Autodesk Inventor part; units mm, degrees
ref_plane "YZ Plane" through (0, 0, 0) normal (1, 0, 0) x (0, 1, 0)
ref_plane "XZ Plane" through (0, 0, 0) normal (0, 1, 0) x (-1, 0, 0)
ref_plane "XY Plane" through (0, 0, 0) normal (0, 0, 1) x (1, 0, 0)
sketch "Sketch1" plane through (0, 0, 0) normal (0, 0, 1) x (1, 0, 0)
  line L0 (-129.1, 49.6) -> (111.9, 49.6)
  line L1 (111.9, 49.6) -> (111.9, -75.4)
  line L2 (111.9, -75.4) -> (-129.1, -75.4)
  line L3 (-129.1, -75.4) -> (-129.1, 49.6)
  line L4 (-116.8, -67) -> (-68.1, -67)
  line L5 (-45.7, -67) -> (3, -67)
  line L6 (3, 18.4) -> (-45.7, 18.4)
  line L7 (-116.8, 18.5) -> (-68.1, 18.5)
  line L8 (-120.7, 14.5) -> (-120.7, -63.1)
  line L9 (-120.7, -67) -> (7.3759, -67) construction
  line L10 (7.3759, -67) -> (7.3759, 18.4) construction
  line L11 (7.3759, 18.4) -> (-120.7, 18.4) construction
  line L12 (-120.7, 18.4) -> (-120.7, -67) construction
  line L13 (4.7803, -64.4044) -> (-118.1044, -64.4044)
  line L14 (-118.1044, -64.4044) -> (-118.1044, 15.8044)
  line L15 (-118.1044, 15.8044) -> (4.7803, 15.8044)
  line L16 (4.7803, 15.8044) -> (4.7803, -64.4044)
  line L17 (-129.1, -55.4) -> (-129.1, -65.4)
  line L18 (-129.1, -75.4) -> (-119.1, -75.4) construction
  line L19 (111.9, -72.4764) -> (111.9, -32.5764) construction
  dimension "d78" = 0
extrude "Extrusion1" add sketch "Sketch1" along normal blind 2
sketch "Sketch10" plane through (0, 0, 0) normal (0, 0, -1) x (-1, 0, 0)
  line L0 (129.1, 49.6) -> (-111.9, 49.6)
  line L1 (-111.9, 49.6) -> (-111.9, -75.4)
  line L2 (-111.9, -75.4) -> (129.1, -75.4)
  line L3 (129.1, -75.4) -> (129.1, 49.6)
  line L4 (-104.9, -68.4) -> (-104.9, 42.6)
  line L5 (-104.9, 42.6) -> (122.1, 42.6)
  line L6 (122.1, 42.6) -> (122.1, -68.4)
  line L7 (122.1, -68.4) -> (-104.9, -68.4)
  line L8 (-3, 18.4) -> (45.7, 18.4)
  line L9 (-6.9, -63.1) -> (-6.9, 14.5)
  line L10 (122.1, 42.6) -> (-104.9, 42.6)
  line L11 (-104.9, 42.6) -> (-104.9, 20.8044)
  line L12 (-104.9, 20.8044) -> (122.1, 20.8044)
  line L13 (122.1, 20.8044) -> (122.1, 42.6)
  line L14 (-104.9, 20.8044) -> (-10.7803, 20.8044)
  line L15 (-10.7803, 20.8044) -> (-10.7803, -68.4)
  line L16 (-10.7803, -68.4) -> (-104.9, -68.4)
  line L17 (-104.9, -68.4) -> (-104.9, 20.8044)
  line L18 (-4.7803, 15.8044) -> (118.1044, 15.8044)
  line L19 (-104.9, 20.8044) -> (-12.287, 20.8044)
  line L20 (-12.287, 20.8044) -> (-12.287, -68.4)
  line L21 (-12.287, -68.4) -> (-104.9, -68.4)
  line L22 (-104.9, -68.4) -> (-104.9, 20.8044)
  line L23 (-4.7803, -64.4044) -> (-4.7803, 15.8044)
  point P0 (0, 0)
  dimension "d73" = 7
  dimension "d86" = 5
  dimension "d87" = 6
extrude "Extrusion7" add sketch "Sketch10" along normal blind 4 contours L3 L2 L1 L0 | L4 L12 L20 L7 | L4 L5 L6 L12 | L20 L12 L15 L7
sketch "Sketch11" plane through (0, 0, -4) normal (0, 0, -1) x (-1, 0, 0)
  circle A0 centre (124.1, -70.4) radius 1.9
  circle A1 centre (124.1, 44.6) radius 1.9
  circle A2 centre (-106.9, -15.5764) radius 3.5
  point P0 (-107.1551, -15.9364)
hole "Hole5" at (-124.1, 44.6, -4) at (-124.1, -70.4, -4) at (106.9, -15.5764, -4) direction (0, 0, 1) diameter 4.3 depth 8 tip angle 118
fillet "Fillet2" radius 2 4 edges at (10.7803, 20.8044, -2) (10.7803, -68.4, -2) (-122.1, 20.8044, -2) (-122.1, -68.4, -2)
sketch "Sketch12" plane through (0, 0, -4) normal (0, 0, -1) x (-1, 0, 0)
  circle A0 centre (124.1, -70.4) radius 2.15
  circle A1 centre (124.1, 44.6) radius 2.15
  circle A2 centre (-106.9, -15.5764) radius 2.15
  line L0 (129.1, -75.4) -> (129.1, 49.6)
  line L1 (129.1, 49.6) -> (-111.9, 49.6)
  line L2 (-111.9, 49.6) -> (-111.9, -75.4)
  line L3 (-111.9, -75.4) -> (129.1, -75.4)
  arc A3 (-8.7803, 20.8044) -> (-10.7803, 18.8044) centre (-8.7803, 18.8044) ccw
  line L4 (120.1, 20.8044) -> (-8.7803, 20.8044)
  arc A4 (122.1, 18.8044) -> (120.1, 20.8044) centre (120.1, 18.8044) ccw
  line L5 (122.1, 18.8044) -> (122.1, -66.4)
  arc A5 (120.1, -68.4) -> (122.1, -66.4) centre (120.1, -66.4) ccw
  line L6 (120.1, -68.4) -> (-8.7803, -68.4)
  arc A6 (-10.7803, -66.4) -> (-8.7803, -68.4) centre (-8.7803, -66.4) ccw
  line L7 (-10.7803, 18.8044) -> (-10.7803, -66.4)
  line L8 (7.5087, 20.8044) -> (25.978, 14.0821)
  line L9 (25.978, 14.0821) -> (27.478, 14.0821)
  line L10 (27.478, 14.0821) -> (27.478, 15.1324)
  line L11 (27.478, 15.1324) -> (11.8945, 20.8044)
  line L12 (120.1, 20.8044) -> (-8.7803, 20.8044)
  line L13 (-10.7803, 18.8044) -> (-10.7803, -66.4)
  line L14 (120.1, 20.8044) -> (-8.7803, 20.8044)
  point P0 (0, 0)
  dimension "d89" = 1.5
  dimension "d90" = 1.5
  dimension "d91" = 160
extrude "Extrusion9" add sketch "Sketch12" against normal blind 3 contours L4 L11 L10 L9 L8
pattern_linear "Rectangular Pattern2" count 3 spacing 30 along (-1, 0, 0) of "Extrusion9"
sketch "Sketch13" plane through (0, 0, 2) normal (0, 0, 1) x (1, 0, 0)
  line L0 (-85.978, 14.0821) -> (-67.5087, 20.8044)
  line L1 (-71.8945, 20.8044) -> (-87.478, 15.1324)
  line L2 (-55.978, 14.0821) -> (-37.5087, 20.8044)
  line L3 (-41.8945, 20.8044) -> (-57.478, 15.1324)
  line L4 (-25.978, 14.0821) -> (-7.5087, 20.8044)
  line L5 (-11.8945, 20.8044) -> (-27.478, 15.1324)
  line L6 (-116.8, 18.4) -> (3, 18.4)
  line L7 (-87.9063, 8.4273) -> (-67.5087, 8.4273)
  line L8 (-67.5087, 8.4273) -> (-67.5087, 18.4)
  line L9 (-67.5087, 18.4) -> (-87.9063, 18.4)
  line L10 (-87.9063, 18.4) -> (-87.9063, 8.4273)
  line L11 (-57.955, 8.4273) -> (-37.5087, 8.4273)
  line L12 (-37.5087, 8.4273) -> (-37.5087, 18.4)
  line L13 (-37.5087, 18.4) -> (-57.955, 18.4)
  line L14 (-57.955, 18.4) -> (-57.955, 8.4273)
  line L15 (-27.478, 8.4273) -> (-7.5087, 8.4273)
  line L16 (-7.5087, 8.4273) -> (-7.5087, 18.4)
  line L17 (-7.5087, 18.4) -> (-27.478, 18.4)
  line L18 (-27.478, 18.4) -> (-27.478, 8.4273)
  point P0 (0, 0)
extrude "Extrusion10" cut sketch "Sketch13" against normal blind 3
sketch "Sketch14" plane through (0, 0, -4) normal (0, 0, -1) x (-1, 0, 0)
  circle A0 centre (-92.31, 42.06) radius 1.5875
  circle A1 centre (-41.51, 26.82) radius 1.5875
  circle A2 centre (-93.58, -6.2) radius 1.5875
  circle A3 centre (-41.51, -1.12) radius 1.5875
  circle A4 centre (-86.028, -17.9) radius 1.375
  circle A5 centre (-28.028, -17.9) radius 1.375
  circle A6 centre (-28.028, -66.9) radius 1.375
  circle A7 centre (-86.028, -66.9) radius 1.375
  point P0 (0, 0)
sketch "Sketch15" plane through (0, 0, -4) normal (0, 0, -1) x (-1, 0, 0)
  point P0 (0, 0)
  point P1 (-92.2892, 42.0744)
  point P2 (-41.6093, 26.9941)
  point P3 (-41.6093, -0.9417)
  point P4 (-28.0946, -17.835)
  point P5 (-28.0122, -66.8668)
  point P6 (-86.1911, -66.8668)
  point P7 (-86.1911, -17.9174)
  point P8 (-93.6077, -6.3805)
hole "Hole6" at (92.2892, 42.0744, -4) at (41.6093, 26.9941, -4) at (41.6093, -0.9417, -4) at (28.0946, -17.835, -4) at (28.0122, -66.8668, -4) at (86.1911, -66.8668, -4) at (86.1911, -17.9174, -4) at (93.6077, -6.3805, -4) direction (0, 0, 1) diameter 2.8 end through all
properties part number "04_OPENTRONS_Microscope_wellplate_base"
Geometry: final body of the model. Coordinates: model frame, mm. A direction names the side the tool comes from. Round coordinates to 2 decimals unless told otherwise and drop trailing zeros. Loops run counter-clockwise (first coordinate to the right, second up) from the corner with the lowest first, then second, coordinate; pieces in that order, holes last.
Q1. Pull-direction query (Y, two-part tool) for faces 1 (the flat face through (-129.1, -14, -1)), 2 (the flat face through (-49.795, 17.929, -2.521)), 3 (the flat face through (-7, -75.4, -1)); classes: released by +Y, released by -Y, zero draft, split by the parting line, or undercut.
Q2. Material intervals for L1, parallel to X at y = -22.5, z = -3.15; L2, parallel to Y at x = -100.5, z = -1.1; L3, parallel to X at y = -45, z = 0.35, sorted ascending.
Q3. Section A-A on y = -34.5. Return loops of the section in (x, z).
Q4. Section B-B on x = -105.5. Return loops of the section in (y, z), plus the area to 3 significant figures.
Q5. Section C-C on x = -47. Return loops of the section in (y, z).
Q6. Access query for faces 4 (the cylindrical face through (-126.23, 44.32, -0.96)), 5 (the flat face through (-78, 18, -1)), 6 (the flat face through (-46.61, 17.49, -2.52)). Directions: +Z, -Z, +X, -X, +Y, -Y. A direction counts if a zero-diameter tool reaches every point of the face in a straight line with its end or side. Return the directions, or none.
Q7. Section D-D on z = -2.35. State how many separate pieces and enclosed holes the cut face has, plus the area to 3 significant figures.
Evaluation:
1. face 1: zero draft
1. face 2: undercut
1. face 3: released by -Y
2. L1: x = -129.1 to -122.1, 10.78 to 111.9
2. L2: y = -75.4 to -68.4, 20.8 to 49.6
2. L3: x = -129.1 to -118.1, 4.78 to 111.9
3. outline: (-129.1, -4) - (-122.1, -4) - (-122.1, 0) - (-118.1, 0) - (-118.1, 2) - (-129.1, 2) - close; (4.78, 0) - (10.78, 0) - (10.78, -4) - (111.9, -4) - (111.9, 2) - (4.78, 2) - close
4. outline: (-75.4, -4) - (-68.4, -4) - (-68.4, 0) - (-64.4, 0) - (-64.4, 2) - (-75.4, 2) - close; (15.8, 0) - (20.8, 0) - (20.8, -4) - (49.6, -4) - (49.6, 2) - (15.8, 2) - close
4. area: 233 mm2
5. outline: (-75.4, -4) - (-68.4, -4) - (-68.4, 0) - (-64.4, 0) - (-64.4, 2) - (-75.4, 2) - close; (17.35, -4) - (18.95, -4) - (18.95, -1) - (17.35, -1) - close; (18.4, 0) - (20.8, 0) - (20.8, -4) - (49.6, -4) - (49.6, 2) - (18.4, 2) - close
6. face 4: +Z, -Z
6. face 5: none
6. face 6: -Z
7. separate pieces: 1
7. enclosed holes: 12
7. area: 18,300 mm2
